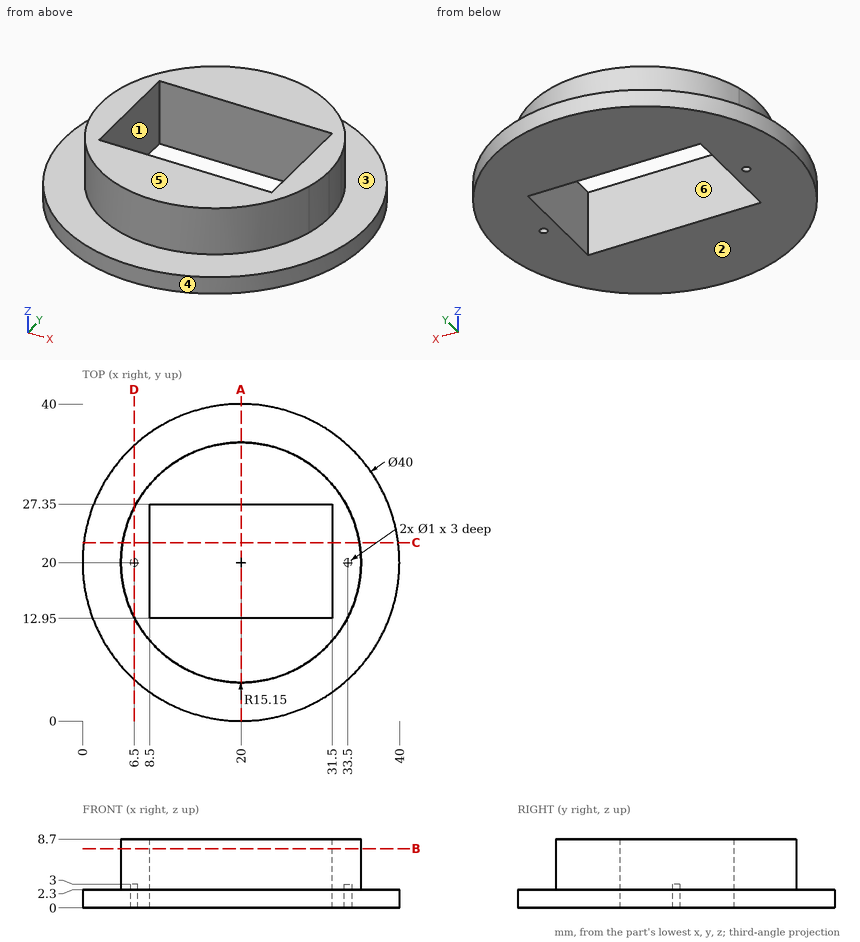
Can you work these out from the drawing? Everything is in mm from the part's minimum corner. A direction names the side the tool comes from. Coordinates: 2 decimals unless noted, no trailing zeros. Loops run counter-clockwise (first coordinate to the right, second up) from the corner with the lowest first, then second, coordinate; pieces in that order, holes last.
1. Imagine slicing it at C-C, the plane y = 22.5. Please give me the cut outline in (x, z).
2. If we mould it in two halves opening along Y, with no side actions, what happens to the marked faces 4, 5 and 6? For each: pulls with the +Y half, pulls with the -Y half, needs draft (parallel to the pull), parting line crosses it, or undercut.
3. Imagine slicing it at D-D, the plane x = 6.5. Please give me the cut outline in (y, z), and give its area (3 significant figures).
4. I need wall thicknesses on L1, parallel to X at y = 20.5, z = 5.5; L2, parallel to Y at x = 9, z = 2.5; L3, parallel to Z at x = 11.5, y = 34.5. Which ranges of each line are inside material? Lowest first, please.
5. For the marked faces 1, 2 and 3, which set-ups out of +Z, -Z, +X, -X, +Y, -Y let a thin tool reach every point of the face, with its end or its side?
6. Imagine slicing it at B-B, the plane z = 7.5. Please give me the cut outline in (x, y).
7. Imagine slicing it at A-A, the plane x = 20. Please give me the cut outline in (y, z).
8. For P1, Ø4, axis at x = 26.5, y = 27.5, coming from the -Z side; P2, Ø4, axis at x = 29, z = 4, coming from the -Y side; P3, Ø0.8, axis at x = 33.5, y = 20, coming from the -Z side; P4, Ø4.5, axis at x = 19, z = 6.5, coming from the +Y side, each with a flat end and sliding along its axis, tell me the tip position at first contact or that it passes through.
Taken from the geometry:
1. outline: (0.16, 0) - (8.5, 0) - (8.5, 8.7) - (5.06, 8.7) - (5.06, 2.3) - (0.16, 2.3) - close; (31.5, 0) - (39.84, 0) - (39.84, 2.3) - (34.94, 2.3) - (34.94, 8.7) - (31.5, 8.7) - close
2. face 4: parting line crosses it
2. face 5: needs draft
2. face 6: undercut
3. outline: (5.24, 0) - (19.5, 0) - (19.5, 3) - (20.5, 3) - (20.5, 0) - (34.76, 0) - (34.76, 2.3) - (26.88, 2.3) - (26.88, 8.7) - (13.12, 8.7) - (13.12, 2.3) - (5.24, 2.3) - close
3. area: 153 mm2
4. L1: x = 4.86 to 8.5, 31.5 to 35.14
4. L2: y = 9.58 to 12.95, 27.35 to 30.42
4. L3: z = 0 to 2.3
5. face 1: +Z, -Z
5. face 2: -Z, +X, -X, +Y, -Y
5. face 3: +Z
6. outline: circle Ø30.3 at (20, 20); hole (8.5, 12.95) - (31.5, 12.95) - (31.5, 27.35) - (8.5, 27.35) - close
7. outline: (0, 0) - (12.95, 0) - (12.95, 8.7) - (4.85, 8.7) - (4.85, 2.3) - (0, 2.3) - close; (27.35, 0) - (40, 0) - (40, 2.3) - (35.15, 2.3) - (35.15, 8.7) - (27.35, 8.7) - close
8. P1: stops at z = 0
8. P2: stops at y = 1.65
8. P3: stops at z = 3
8. P4: stops at y = 35.15
